Autodesk Fusion 360 part; units mm, degrees
sketch "ValveAdapterBase" plane through (0, 0, 0) normal (1, 0, 0) x (0, 1, 0) in component "ValveHalterung"
  line L0 (-15, 15) -> (15, 15) construction
  line L1 (15, 15) -> (15, -15) construction
  line L2 (15, -15) -> (-15, -15) construction
  line L3 (-15, -15) -> (-15, 15) construction
  line L4 (-15, 15) -> (15, -15) construction
  line L5 (15, 15) -> (-15, -15) construction
  circle A0 centre (15, 15) radius 1.7
  circle A1 centre (15, -15) radius 1.7
  circle A2 centre (-15, -15) radius 1.7
  circle A3 centre (-15, 15) radius 1.7
  line L6 (-20, 20) -> (20, 20)
  line L7 (20, 20) -> (20, -20)
  line L8 (20, -20) -> (-20, -20)
  line L9 (-20, -20) -> (-20, 20)
  line L10 (-20, 20) -> (20, -20) construction
  line L11 (20, 20) -> (-20, -20) construction
  line L12 (-16.5877, 17.75) -> (-18.1754, 15)
  line L13 (-18.1754, 15) -> (-16.5877, 12.25)
  line L14 (-16.5877, 12.25) -> (-13.4123, 12.25)
  line L15 (-13.4123, 12.25) -> (-11.8246, 15)
  line L16 (-11.8246, 15) -> (-13.4123, 17.75)
  line L17 (-13.4123, 17.75) -> (-16.5877, 17.75)
  line L18 (0, 33) -> (0, -35) construction
  line L19 (41, 0) -> (-42, 0) construction
  line L20 (11.8246, 15) -> (13.4123, 17.75)
  line L21 (13.4123, 17.75) -> (16.5877, 17.75)
  line L22 (16.5877, 17.75) -> (18.1754, 15)
  line L23 (18.1754, 15) -> (16.5877, 12.25)
  line L24 (13.4123, 12.25) -> (11.8246, 15)
  line L25 (16.5877, 12.25) -> (13.4123, 12.25)
  line L26 (-18.1754, -15) -> (-16.5877, -12.25)
  line L27 (-16.5877, -12.25) -> (-13.4123, -12.25)
  line L28 (-13.4123, -12.25) -> (-11.8246, -15)
  line L29 (-11.8246, -15) -> (-13.4123, -17.75)
  line L30 (-16.5877, -17.75) -> (-18.1754, -15)
  line L31 (-13.4123, -17.75) -> (-16.5877, -17.75)
  line L32 (18.1754, -15) -> (16.5877, -12.25)
  line L33 (16.5877, -12.25) -> (13.4123, -12.25)
  line L34 (13.4123, -12.25) -> (11.8246, -15)
  line L35 (11.8246, -15) -> (13.4123, -17.75)
  line L36 (16.5877, -17.75) -> (18.1754, -15)
  line L37 (13.4123, -17.75) -> (16.5877, -17.75)
  circle A4 centre (7.3158, 9.4632) radius 2.1
  point P0 (-15, 15)
  dimension "d4" = 30
  dimension "d7" = 3.4
  dimension "d8" = 3.4
  dimension "d9" = 3.4
  dimension "d10" = 3.4
  dimension "d12" = 40
  dimension "d17" = 2.75
  dimension "d22" = 4.2
extrude "Extrude1" add sketch "ValveAdapterBase" against normal blind 8 contours L6 L7 L8 L9 | L12 L13 L14 L15 L16 L17 | L20 L21 L22 L23 L24 L25 | L26 L27 L28 L29 L30 L31 | L32 L33 L34 L35 L36 L37 | A4 in component "ValveHalterung"
extrude "Extrude2" cut sketch "ValveAdapterBase" against normal blind 3 contours L12 L13 L14 L15 L16 L17 | L20 L21 L22 L23 L24 L25 | L26 L27 L28 L29 L30 L31 | L32 L33 L34 L35 L36 L37 in component "ValveHalterung"
sketch "ValveAdapterScrews" plane through (-8, 0, 0) normal (-1, 0, 0) x (0, -1, 0) in component "ValveHalterung"
  circle A0 centre (-15, 15) radius 1.7
  circle A1 centre (15, 15) radius 1.7
  circle A2 centre (-15, -15) radius 1.7
  circle A3 centre (15, -15) radius 1.7
  line L0 (-20, -20) -> (20, -20)
  line L1 (20, -20) -> (20, 20)
  line L2 (20, 20) -> (-20, 20)
  line L3 (-20, 20) -> (-20, -20)
  line L4 (-15, 11) -> (15, 11) construction
  line L5 (15, 11) -> (15, -11) construction
  line L6 (15, -11) -> (-15, -11) construction
  line L7 (-15, -11) -> (-15, 11) construction
  line L8 (-15, 11) -> (15, -11) construction
  line L9 (15, 11) -> (-15, -11) construction
  circle A4 centre (9.7, 7.1) radius 2.1
  line L10 (11.8, 7.1) -> (11.8, 11) construction
  line L11 (9.7, 9.2) -> (15, 9.2) construction
  line L12 (31, -0.4) -> (-34, -0.4) construction
  circle A5 centre (9.7, -7.9) radius 2.1
  circle A6 centre (9.7, 7.1) radius 4.5
  circle A7 centre (9.7, -7.9) radius 4.5
  dimension "d35" = 30
  dimension "d36" = 22
  dimension "d37" = 4.2
  dimension "d38" = 3.2
  dimension "d39" = 1.8
  dimension "d42" = 9
  dimension "d47" = 15
extrude "Extrude3" cut sketch "ValveAdapterScrews" against normal up to surface (8 mm away) contours A4 | A5 in component "ValveHalterung"
extrude "Extrude4" cut sketch "ValveAdapterScrews" against normal blind 4.5 contours A6 | A7 in component "ValveHalterung"
chamfer "Chamfer1" distance 2 angle 45 4 edges at (-4, -20, 20) (-4, 20, 20) (-4, -20, -20) (-4, 20, -20) in component "ValveHalterung"
component "ValveHalterung" placed x (1, 0, 0) y (0, 1, 0) z (0, 0, 1) at (0, 0, 0)
equation "Staging_Plate_Spacing = 30 mm"
equation "d4 = Staging_Plate_Spacing"
equation "M3_Screw_Diameter = 3.4 mm"
equation "d7 = M3_Screw_Diameter"
equation "d8 = M3_Screw_Diameter"
equation "d9 = M3_Screw_Diameter"
equation "d10 = M3_Screw_Diameter"
equation "Outer_Edge = 40 mm"
equation "d12 = Outer_Edge"
equation "M3_Nut_Edge = 5.5 mm"
equation "d17 = M3_Nut_Edge / 2"
equation "M3_Nut_Extrusion = 3 mm"
equation "d19 = -M3_Nut_Extrusion"
equation "Valve_Screw_Diameter = 4.2 mm"
equation "d22 = Valve_Screw_Diameter"
equation "d37 = Valve_Screw_Diameter"
equation "d42 = Valve_Screw_Head_Diameter"
equation "Valve_Screw_Head_Diameter = 9 mm"
CAD build for the part. Positions are in the model's coordinates, mm. A direction names the side the tool comes from. Give positions to 0.01 mm unless a question says otherwise; leave off trailing zeros. Order: outer loops, then holes, each group sorted by start corner. A loop starts at its lowest first (then second) coordinate and runs counter-clockwise, first axis right, second up.
(1) Flat gauge pins, fed straight in: pin 1 (5.5 mm diameter, centred on y = -9.7, z = 7.1, fed in from +X); pin 2 (4.5 mm diameter, centred on y = -10.5, z = 7.5, fed in from -X); pin 3 (1.6 mm diameter, centred on y = -15.5, z = 15, fed in from +X). Where does each tip first touch, or does it go through?
(2) Mould opens along Y. For faces 4 (the flat face through (-4, 19, -19)), 5 (the flat face through (-1.48, 12.61, -16.36)), 6 (the flat face through (0, 0, 0)) say: released by +Y, released by -Y, zero draft, split by the parting line, or undercut.
(3) Saw through at A-A, the plane y = -15. Give the cut face in (x, z), then the cut area to 3 significant figures.
(4) Saw through at D-D, the plane z = 3.5. Give the cut face in (x, y), then the cut area to 3 significant figures.
(5) Tool access for faces 1 (the flat face through (-3, 16.4, -13.7)), 2 (the cylindrical face through (-5.78, -13.86, -9.62)), 3 (the cylindrical face through (-5.46, -13.38, -14.49)): list every direction of +Z, -Z, +X, -X, +Y, -Y with a clear straight run to the whole face (end or side of a thin tool).
(6) Drill centre lines: L1, parallel to Z at x = -4.1, y = -15; L2, parallel to Z at x = -1.5, y = -9.7; L3, parallel to Y at x = -0.5, z = -14. Where is each one in solid material? Low to high.
(7) Saw through at B-B, the plane x = -1.25. State how many separate pieces and enclosed holes the cut face has, then the cut area to 3 significant figures.
(8) Saw through at C-C, the plane z = -7.9. Give the cut face in (x, y), then the cut area to 3 significant figures.
Results found:
1. pin 1: stops at x = 0
1. pin 2: stops at x = -3.5
1. pin 3: passes through
2. face 4: released by +Y
2. face 5: undercut
2. face 6: zero draft
3. outline: (-8, -20) - (0, -20) - (0, -17.75) - (-3, -17.75) - (-3, -16.7) - (-8, -16.7) - close; (-8, -13.3) - (-3, -13.3) - (-3, -12.25) - (0, -12.25) - (0, 12.25) - (-3, 12.25) - (-3, 13.3) - (-8, 13.3) - close; (-8, 16.7) - (-3, 16.7) - (-3, 17.75) - (0, 17.75) - (0, 20) - (-8, 20) - close
3. area: 253 mm2
4. outline: (-8, -20) - (0, -20) - (0, 20) - (-8, 20) - (-8, -7) - (-3.5, -7) - (-3.5, -12.4) - (-8, -12.4) - close
4. area: 296 mm2
5. face 1: +X
5. face 2: -X
5. face 3: +X, -X
6. L1: z = -20 to -16.7, -13.3 to 13.3, 16.7 to 20
6. L2: z = -20 to -10, -5.8 to 5, 9.2 to 20
6. L3: y = -20 to -17.6, -12.4 to 12.4, 17.6 to 20
7. separate pieces: 1
7. enclosed holes: 6
7. area: 1,460 mm2
8. outline: (-8, -20) - (0, -20) - (0, -11.8) - (-3.5, -11.8) - (-3.5, -14.2) - (-8, -14.2) - close; (-8, -5.2) - (-3.5, -5.2) - (-3.5, -7.6) - (0, -7.6) - (0, 20) - (-8, 20) - close
8. area: 265 mm2
